Autodesk Fusion 360 part; units mm, degrees
sketch "Sketch1" plane through (0, 0, 0) normal (0, 0, 1) x (1, 0, 0)
  line L0 (-50, 50) -> (35, 50)
  line L1 (35, 50) -> (35, -5)
  line L2 (35, -5) -> (-50, -5)
  line L3 (-50, -5) -> (-50, 50)
extrude "Extrude1" add sketch "Sketch1" along normal blind 19
extrude "Extrude2" cut 1 faces at (-21.6667, 31.6667, 19) along direction (0, 0, -1) blind 1
sketch "Sketch2" plane through (0, 0, 0) normal (0, 0, 1) x (1, 0, 0)
  line L0 (35, 50) -> (55, 50)
  line L1 (55, 50) -> (55, -5)
  line L2 (55, -5) -> (35, -5)
  line L3 (35, -5) -> (35, 50)
  line L4 (-50, 50) -> (-70, 50)
  line L5 (-70, 50) -> (-70, -5)
  line L6 (-70, -5) -> (-50, -5)
  line L7 (-50, -5) -> (-50, 50)
extrude "Extrude3" add sketch "Sketch2" along normal blind 11
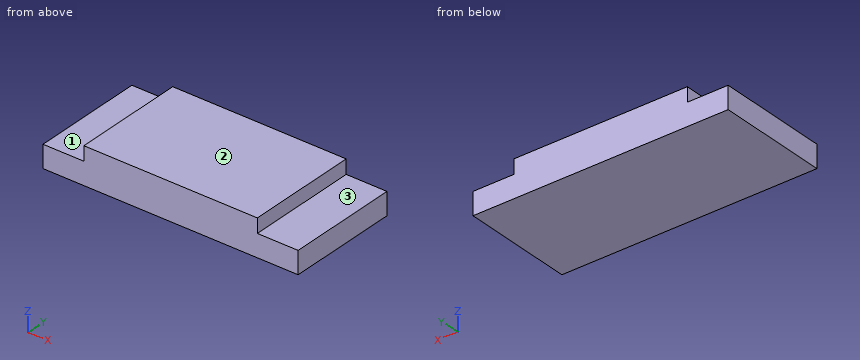
The model under review builds one solid part; all positions refer to its coordinate system, in mm. Face numbers are marked on the shaded views. A direction names the side the tool comes from. Give positions to 0.01 mm unless a question says otherwise; leave off trailing zeros. Loops run counter-clockwise (first coordinate to the right, second up) from the corner with the lowest first, then second, coordinate; pieces in that order, holes last. Notation, with made-up numbers: (63.5, 75) -> (78.5, 75) arc R23 cw to (78.5, 108) -> close; hole circle Ø6 at (77, -29.75). An arc over 180 degrees is marked (long way). Write each question's results on one line, items separated by ' | '.
1) For line 1 along Z through (x, y) = (-50.5, 43.5); line 2 along X through (y, z) = (2.5, 15), list the stretches that pass through material, from the lowest coordinate up. Write a range as from..to.
Conclusion:
line 1: z = 0..11 | line 2: x = -50..35
2) Tool access review of the marked faces 1, 2 and 3: name each direction out of +Z, -Z, +X, -X, +Y, -Y from which nothing blocks a thin tool from reaching the whole face with its end or side.
Conclusion:
face 1: +Z, -X, +Y, -Y | face 2: +Z, +X, -X, +Y, -Y | face 3: +Z, +X, +Y, -Y
3) Take a section at A-A, the plane y = 29.5. Give the boundary of the cut face in (x, z), plus the area to 3 significant figures.
Conclusion:
outline: (-70, 0) -> (55, 0) -> (55, 11) -> (35, 11) -> (35, 18) -> (-50, 18) -> (-50, 11) -> (-70, 11) -> close | area: 1,970 mm^2
4) Take a section at B-B, the plane z = 14.75. Give the boundary of the cut face in (x, y).
Conclusion:
outline: (-50, -5) -> (35, -5) -> (35, 50) -> (-50, 50) -> close
5) Insertion check: pin 1 Ø6 at (x, y) = (-56, 9) entering from +Z; pin 2 Ø2 at (y, z) = (10.5, 16) entering from +X. Each pin has a flat end and moves straight along its axis. Give the tip position at first contact, or say it passes through.
Conclusion:
pin 1: stops at z = 11 | pin 2: stops at x = 35
